Could you check a few things on this model? Use its own coordinates, in mm. A direction names the side the tool comes from. Give positions to 0.01 mm unless a question says otherwise; leave off trailing zeros. Write each loop counter-clockwise with the first axis right and the second up, starting at its lowest first coordinate (ties: lowest second). Pieces come first, ordered by that corner, then holes. Notation, with made-up numbers: (84.25, 36.5) - (143.25, 36.5) arc R19 cw to (143.25, 66.5) - close; hole circle Ø11 at (69, -6). An arc over 180 degrees is marked (long way). Answer in a Markdown table with one row per item.
from build123d import *

# Parameters (mm, degrees)
ESQUISSE1_R        = 1.75
BOSS_EXTRU_1_DEPTH = 2


with BuildPart() as part:
    # Esquisse1 → Boss.-Extru.1 (new body, symmetric)
    with BuildSketch(Plane.XY):
        with BuildLine():
            ThreePointArc((30.75, -4), (34.75, 0), (30.75, 4))
            Line((30.75, 4), (11.409123542, 4))
            ThreePointArc((11.409123542, 4), (11.194344337, 4.566700654), (10.951436862, 5.12192646))
            ThreePointArc((10.951436862, 5.12192646), (12.008090957, 5.965388247), (12.82210701, 7.044889767))
            ThreePointArc((12.82210701, 7.044889767), (12.669951657, 7.315), (12.51210701, 7.581825517))
            ThreePointArc((12.51210701, 7.581825517), (11.170223244, 7.416617696), (9.911436862, 6.9232593))
            ThreePointArc((9.911436862, 6.9232593), (9.591641884, 7.359925677), (9.252623584, 7.781841479))
            ThreePointArc((9.252623584, 7.781841479), (10.05496909, 8.870045207), (10.561852666, 10.123446462))
            ThreePointArc((10.561852666, 10.123446462), (10.344972209, 10.344972209), (10.123446462, 10.561852666))
            ThreePointArc((10.123446462, 10.561852666), (8.870045207, 10.05496909), (7.781841479, 9.252623584))
            ThreePointArc((7.781841479, 9.252623584), (7.359925677, 9.591641884), (6.9232593, 9.911436862))
            ThreePointArc((6.9232593, 9.911436862), (7.416617696, 11.170223244), (7.581825517, 12.51210701))
            ThreePointArc((7.581825517, 12.51210701), (7.315, 12.669951657), (7.044889767, 12.82210701))
            ThreePointArc((7.044889767, 12.82210701), (5.965388247, 12.008090957), (5.12192646, 10.951436862))
            ThreePointArc((5.12192646, 10.951436862), (4.626642697, 11.169703548), (4.122086336, 11.365584201))
            ThreePointArc((4.122086336, 11.365584201), (4.272836063, 12.709169027), (4.085109489, 14.048088143))
            ThreePointArc((4.085109489, 14.048088143), (3.78652263, 14.131494839), (3.486235477, 14.208555951))
            ThreePointArc((3.486235477, 14.208555951), (2.654199937, 13.14288127), (2.112960617, 11.903927815))
            ThreePointArc((2.112960617, 11.903927815), (1.578061664, 11.986568374), (1.04, 12.04518576))
            ThreePointArc((1.04, 12.04518576), (0.837867713, 13.382005944), (0.31, 14.626715284))
            ThreePointArc((0.31, 14.626715284), (0, 14.63), (-0.31, 14.626715284))
            ThreePointArc((-0.31, 14.626715284), (-0.837867713, 13.382005944), (-1.04, 12.04518576))
            ThreePointArc((-1.04, 12.04518576), (-1.578061664, 11.986568374), (-2.112960617, 11.903927815))
            ThreePointArc((-2.112960617, 11.903927815), (-2.654199937, 13.14288127), (-3.486235477, 14.208555951))
            ThreePointArc((-3.486235477, 14.208555951), (-3.78652263, 14.131494839), (-4.085109489, 14.048088143))
            ThreePointArc((-4.085109489, 14.048088143), (-4.272836063, 12.709169027), (-4.122086336, 11.365584201))
            ThreePointArc((-4.122086336, 11.365584201), (-4.626642697, 11.169703548), (-5.12192646, 10.951436862))
            ThreePointArc((-5.12192646, 10.951436862), (-5.965388247, 12.008090957), (-7.044889767, 12.82210701))
            ThreePointArc((-7.044889767, 12.82210701), (-7.315, 12.669951657), (-7.581825517, 12.51210701))
            ThreePointArc((-7.581825517, 12.51210701), (-7.416617696, 11.170223244), (-6.9232593, 9.911436862))
            ThreePointArc((-6.9232593, 9.911436862), (-7.359925677, 9.591641884), (-7.781841479, 9.252623584))
            ThreePointArc((-7.781841479, 9.252623584), (-8.870045207, 10.05496909), (-10.123446462, 10.561852666))
            ThreePointArc((-10.123446462, 10.561852666), (-10.344972209, 10.344972209), (-10.561852666, 10.123446462))
            ThreePointArc((-10.561852666, 10.123446462), (-10.05496909, 8.870045207), (-9.252623584, 7.781841479))
            ThreePointArc((-9.252623584, 7.781841479), (-9.591641884, 7.359925677), (-9.911436862, 6.9232593))
            ThreePointArc((-9.911436862, 6.9232593), (-11.170223244, 7.416617696), (-12.51210701, 7.581825517))
            ThreePointArc((-12.51210701, 7.581825517), (-12.669951657, 7.315), (-12.82210701, 7.044889767))
            ThreePointArc((-12.82210701, 7.044889767), (-12.008090957, 5.965388247), (-10.951436862, 5.12192646))
            ThreePointArc((-10.951436862, 5.12192646), (-11.169703548, 4.626642697), (-11.365584201, 4.122086336))
            ThreePointArc((-11.365584201, 4.122086336), (-12.709169027, 4.272836063), (-14.048088143, 4.085109489))
            ThreePointArc((-14.048088143, 4.085109489), (-14.131494839, 3.78652263), (-14.208555951, 3.486235477))
            ThreePointArc((-14.208555951, 3.486235477), (-13.14288127, 2.654199937), (-11.903927815, 2.112960617))
            ThreePointArc((-11.903927815, 2.112960617), (-11.986568374, 1.578061664), (-12.04518576, 1.04))
            ThreePointArc((-12.04518576, 1.04), (-13.382005944, 0.837867713), (-14.626715284, 0.31))
            ThreePointArc((-14.626715284, 0.31), (-14.63, 0), (-14.626715284, -0.31))
            ThreePointArc((-14.626715284, -0.31), (-13.382005944, -0.837867713), (-12.04518576, -1.04))
            ThreePointArc((-12.04518576, -1.04), (-11.986568374, -1.578061664), (-11.903927815, -2.112960617))
            ThreePointArc((-11.903927815, -2.112960617), (-13.14288127, -2.654199937), (-14.208555951, -3.486235477))
            ThreePointArc((-14.208555951, -3.486235477), (-14.131494839, -3.78652263), (-14.048088143, -4.085109489))
            ThreePointArc((-14.048088143, -4.085109489), (-12.709169027, -4.272836063), (-11.365584201, -4.122086336))
            ThreePointArc((-11.365584201, -4.122086336), (0.064808849, -12.089826294), (11.409123542, -4))
            Line((11.409123542, -4), (30.75, -4))
        make_face()
        with Locations((30.75, 0)):
            Circle(ESQUISSE1_R, mode=Mode.SUBTRACT)
        Circle(ESQUISSE1_R, mode=Mode.SUBTRACT)
    extrude(amount=BOSS_EXTRU_1_DEPTH, both=True)


solid = part.part
1) Will these pins go through, and if not, where does the flat tip stop? P1, Ø2, axis at x = 18, z = -0.5, coming from the +Y side; P2, Ø2, axis at x = -3, z = 0.5, coming from the -Y side; P3, Ø2, axis at x = 24, z = 0, coming from the -Y side; P4, Ø3, axis at x = 0, y = 0, coming from the +Z side.
Check values:
| item | result |
|---|---|
| P1 | stops at y = 4 |
| P2 | stops at y = -11.92 |
| P3 | stops at y = -4 |
| P4 | passes through |
2) Imagine slicing it at C-C (y = -3). List the corners of the cut face in (x, z) for me.
Check values:
| item | result |
|---|---|
| outline | (-13.65, -2) - (33.4, -2) - (33.4, 2) - (-13.65, 2) - close |
3) Imagine slicing it at A-A (z = -0.4). State how many separate pieces and enclosed holes the cut face has, then the cut area to 3 significant figures.
Check values:
| item | result |
|---|---|
| separate pieces | 1 |
| enclosed holes | 2 |
| area | 665 mm2 |
4) If I drill on line 1 (Y direction, x = 0, z = -1.3); line 2 (Y direction, x = 30.75, z = -0.3); line 3 (Y direction, x = 25, z = -1.7), over which ranges is the centre line in solid material (lowest first)?
Check values:
| item | result |
|---|---|
| line 1 | y = -12.09 to -1.75, 1.75 to 14.63 |
| line 2 | y = -4 to -1.75, 1.75 to 4 |
| line 3 | y = -4 to 4 |
5) On a 3-axis mill with a long thin cutter (end or side, diameter ignored), from which of +Z, -Z, +X, -X, +Y, -Y can I reach the whole of each face in a straight line? I mean faces 1 (the face through (-0.14, -12.09, 0.03)), 2 (the face through (-11.988, -1.571, 0.028)), 3 (the face through (1.586, 11.986, 0.028)), 4 (the face through (-11.15, 7.41, 0.03)). Say none if no direction works.
Check values:
| item | result |
|---|---|
| face 1 | +Z, -Z, -Y |
| face 2 | +Z, -Z, -X |
| face 3 | +Z, -Z, +Y |
| face 4 | +Z, -Z |
6) Imagine slicing it at B-B (x = 20.5). List the corners of the cut face in (y, z) for me, then the cut area to 3 significant figures.
Check values:
| item | result |
|---|---|
| outline | (-4, -2) - (4, -2) - (4, 2) - (-4, 2) - close |
| area | 32.0 mm2 |
